Part model, mm, in its own coordinate system. Round coordinates to 2 decimals unless told otherwise and drop trailing zeros. Order: outer loops, then holes, each group sorted by start corner. A loop starts at its lowest first (then second) coordinate and runs counter-clockwise, first axis right, second up. Notation, with made-up numbers: M -30,67 L -4,67 A13 cw -4,83 Z; hole C 55.5,36 d3. An arc over 180 degrees is marked long. One line per question, with ' | ' between items.
from build123d import *

# Parameters (mm, degrees)
SKETCH_W           = 30
SKETCH_H           = 30
PAD_DEPTH          = 120
SKETCH001_W        = 8
SKETCH001_H        = 4
POCKET_DEPTH       = 120
POLARPATTERN_COUNT = 4


with BuildPart() as part:
    # Sketch → Pad (new body)
    with BuildSketch(Plane.XY):
        Rectangle(SKETCH_W, SKETCH_H)
    extrude(amount=PAD_DEPTH)

    # Sketch001 (on Face6 of Pad) → Pocket (cut)
    with BuildSketch(Plane.XY.offset(120)):
        with Locations((0, 13)):
            Rectangle(SKETCH001_W, SKETCH001_H)
    pocket = extrude(amount=-POCKET_DEPTH, mode=Mode.SUBTRACT)

    # PolarPattern: Pocket ×4 about axis
    polarpattern_axis = Axis((0, 0, 120), (0, 0, 1))
    for i in range(1, POLARPATTERN_COUNT):
        add(pocket.rotate(polarpattern_axis, i * 360 / POLARPATTERN_COUNT), mode=Mode.SUBTRACT)


solid = part.part
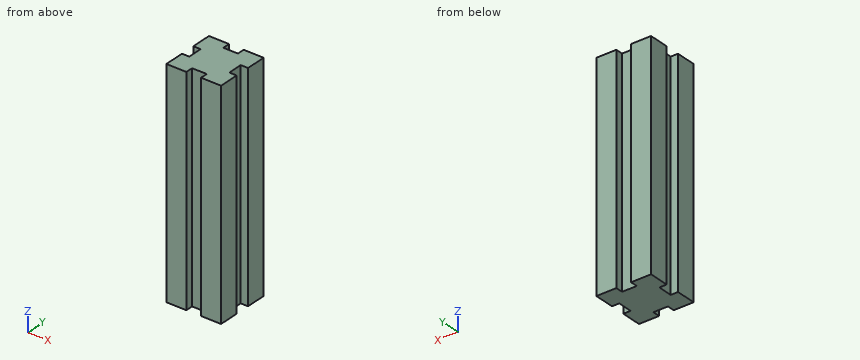
1) Saw through at C-C (x = 2.5). List the corners of the cut face in (y, z), plus the area to 3 significant figures.
The answers:
outline: M -11,0 L 11,0 L 11,120 L -11,120 Z | area: 2,640 mm²
2) Saw through at B-B (z = 63). List the corners of the cut face in (x, y).
The answers:
outline: M -15,-15 L -4,-15 L -4,-11 L 4,-11 L 4,-15 L 15,-15 L 15,-4 L 11,-4 L 11,4 L 15,4 L 15,15 L 4,15 L 4,11 L -4,11 L -4,15 L -15,15 L -15,4 L -11,4 L -11,-4 L -15,-4 Z
3) Probe line 1 (X direction, y = 12.25, z = 81); line 2 (Y direction, x = -1, z = 42). List the from-to ranges inside material, lowest first. Write a range as [from, to].
The answers:
line 1: x = [-15, -4], [4, 15] | line 2: y = [-11, 11]
4) Drop flat-ended pins along their axis: pin 1 (6.5 mm diameter, centred on y = -0.5, z = 77.5, fed in from -X); pin 2 (6.5 mm diameter, centred on x = 0, z = 75, fed in from -Y); pin 3 (2.5 mm diameter, centred on y = -0.5, z = 74, fed in from +X). Give the stop position or say it passes through.
The answers:
pin 1: stops at x = -11 | pin 2: stops at y = -11 | pin 3: stops at x = 11
5) Saw through at A-A (y = 12.25). List the corners of the cut face in (x, z), plus the area to 3 significant figures.
The answers:
outline: M -15,0 L -4,0 L -4,120 L -15,120 Z; M 4,0 L 15,0 L 15,120 L 4,120 Z | area: 2,640 mm²
